Input: part model. Units: mm. Frame: model coordinates. A direction names the side the tool comes from. Coordinates: 2 decimals unless noted, no trailing zeros. Write each loop counter-clockwise with the first axis right and the second up, starting at its lowest first coordinate (ties: lowest second). Pieces come first, ordered by that corner, then holes. Notation, with made-up numbers: M -7,-3.75 L 42,-3.75 A5 cw 42,0.25 Z; hole C -18,82 d8. An arc over 180 degrees is marked long. Use CSV: the item, a comma, the result in double quotes.
```python
from build123d import *

# Parameters (mm, degrees)
SKETCH1_R           = 6.5
BASE_EXTRUDE_DEPTH  = 5
SKETCH2_R           = 4
BOSS_EXTRUDE1_DEPTH = 15
CUT_EXTRUDE1_DEPTH  = 5


with BuildPart() as part:
    # Sketch1 → Base-Extrude (new body)
    with BuildSketch(Plane.XY):
        Circle(SKETCH1_R)
    extrude(amount=BASE_EXTRUDE_DEPTH)

    # Sketch2 → Boss-Extrude1 (add)
    with BuildSketch(Plane(origin=(0, 0, 0), x_dir=(-1, 0, 0), z_dir=(0, 0, -1))):
        Circle(SKETCH2_R)
    extrude(amount=BOSS_EXTRUDE1_DEPTH)

    # Sketch3 → Cut-Extrude1 (cut)
    with BuildSketch(Plane.XY.offset(5)):
        Polygon((0, 3.464101615), (-3, 1.732050808), (-3, -1.732050808), (0, -3.464101615), (3, -1.732050808), (3, 1.732050808), align=None)
    extrude(amount=-CUT_EXTRUDE1_DEPTH, mode=Mode.SUBTRACT)


solid = part.part
```
1. Access query for faces 1 (the flat face through (-1.5, 2.6, 2.5)), 2 (the flat face through (-2, -3, 5)), 3 (the flat face through (3, 3, 0)). Directions: +Z, -Z, +X, -X, +Y, -Y. A direction counts if a zero-diameter tool reaches every point of the face in a straight line with its end or side. Return the directions, or none.
Resolved:
face 1,"+Z"
face 2,"+Z, +X, -X, +Y, -Y"
face 3,"-Z"
2. Section B-B (y = 0). Return loops of the section in (x, z).
Resolved:
outline,"M -6.5,0 L -4,0 L -4,-15 L 4,-15 L 4,0 L 6.5,0 L 6.5,5 L 3,5 L 3,0 L -3,0 L -3,5 L -6.5,5 Z"
3. Contact query for flat-ended pins moving along their axis: pin 1 Ø4 at (y, z) = (2.5, -3) entering from -X; pin 2 Ø1.5 at (x, z) = (-2, -3) entering from +Y; pin 3 Ø5 at (x, z) = (1.5, -12.5) entering from -Y. Output: stop coordinate, or through.
Resolved:
pin 1,"stops at x = -3.97"
pin 2,"stops at y = 3.8"
pin 3,"stops at y = -4"
4. Mould query, pull axis Y, two halves, no side actions, for faces 4 (the flat face through (1.5, 2.6, 2.5)), 5 (the flat face through (0, 0, -15)), 6 (the cylindrical face through (-5.158, -3.955, 2.465)). Classes: pulls with the +Y half, pulls with the -Y half, needs draft (parallel to the pull), parting line crosses it, or undercut.
Resolved:
face 4,"undercut"
face 5,"needs draft"
face 6,"parting line crosses it"
5. Section A-A (z = 2.5). Return loops of the section in (x, y).
Resolved:
outline,"C 0,0 d13; hole M -3,-1.73 L 0,-3.46 L 3,-1.73 L 3,1.73 L 0,3.46 L -3,1.73 Z"
6. Section D-D (z = -5.75). Return loops of the section in (x, y).
Resolved:
outline,"C 0,0 d8"
7. Material intervals for line 1 (X direction, y = -2, z = -8); line 2 (Z direction, x = 3.5, y = -2); line 3 (Z direction, x = -0.25, y = -1), sorted ascending. Write a range as [from, to].
Resolved:
line 1,"x = [-3.46, 3.46]"
line 2,"z = [0, 5]"
line 3,"z = [-15, 0]"
8. Section C-C (x = 0.25). Return loops of the section in (y, z), then the cut area to 3 significant figures.
Resolved:
outline,"M -6.5,0 L -3.99,0 L -3.99,-15 L 3.99,-15 L 3.99,0 L 6.5,0 L 6.5,5 L 3.32,5 L 3.32,0 L -3.32,0 L -3.32,5 L -6.5,5 Z"
area,"152 mm^2"
